```python
from build123d import *

# Parameters (mm, degrees)
EXTRUDE_1_DEPTH     = 3
SKETCH_2_R          = 1.6
SKETCH_2_W          = 1.5
SKETCH_2_H          = 40
CUT_EXTRUDE_1_DEPTH = 160.48040632


with BuildPart() as part:
    # 草图1 → 凸台-拉伸1 (new body)
    with BuildSketch(Plane.XY):
        Polygon((0, 0), (20, 0), (105, -105), (105, -120), (-20, -120), (-20, -105), align=None)
    extrude(amount=EXTRUDE_1_DEPTH)

    # 草图2 → 切除-拉伸1 (cut, through all)
    with BuildSketch(Plane.XY.offset(3)):
        with Locations((5, -5)):
            Circle(SKETCH_2_R)
        with Locations(Location((15, -5, 0), (0, 0, 180))):
            Circle(SKETCH_2_R)
        with Locations((15, -15)):
            Circle(SKETCH_2_R)
        with Locations(Location((5, -15, 0), (0, 0, 180))):
            Circle(SKETCH_2_R)
        with Locations((-15, -116.25)):
            Circle(SKETCH_2_R)
        with Locations(Location((-15, -108.75, 0), (0, 0, 180))):
            Circle(SKETCH_2_R)
        with Locations(Location((-5, -116.25, 0), (0, 0, 180))):
            Circle(SKETCH_2_R)
        with Locations((-5, -108.75)):
            Circle(SKETCH_2_R)
        with Locations(Location((90, -108.75, 0), (0, 0, 180))):
            Circle(SKETCH_2_R)
        with Locations((90, -116.25)):
            Circle(SKETCH_2_R)
        with Locations((100, -108.75)):
            Circle(SKETCH_2_R)
        with Locations(Location((100, -116.25, 0), (0, 0, 180))):
            Circle(SKETCH_2_R)
        with Locations((37.5, -116.25)):
            Circle(SKETCH_2_R)
        with Locations(Location((47.5, -116.25, 0), (0, 0, 180))):
            Circle(SKETCH_2_R)
        with Locations((47.5, -108.75)):
            Circle(SKETCH_2_R)
        with Locations(Location((37.5, -108.75, 0), (0, 0, 180))):
            Circle(SKETCH_2_R)
        with Locations((5, -45)):
            Circle(SKETCH_2_R)
        with Locations(Location((15, -45, 0), (0, 0, 180))):
            Circle(SKETCH_2_R)
        with Locations((15, -55)):
            Circle(SKETCH_2_R)
        with Locations(Location((5, -55, 0), (0, 0, 180))):
            Circle(SKETCH_2_R)
        with Locations(Location((5, -108.75, 0), (0, 0, 180))):
            Circle(SKETCH_2_R)
        with Locations((5, -116.25)):
            Circle(SKETCH_2_R)
        with Locations(Location((15, -116.25, 0), (0, 0, 180))):
            Circle(SKETCH_2_R)
        with Locations((15, -108.75)):
            Circle(SKETCH_2_R)
        with Locations((70, -116.25)):
            Circle(SKETCH_2_R)
        with Locations(Location((80, -116.25, 0), (0, 0, 180))):
            Circle(SKETCH_2_R)
        with Locations(Location((70, -108.75, 0), (0, 0, 180))):
            Circle(SKETCH_2_R)
        with Locations((80, -108.75)):
            Circle(SKETCH_2_R)
        Polygon((-2, -53.255116653), (-2, -102.5), (-11.37997778, -102.5), align=None)
        with Locations((104.25, -100)):
            Rectangle(SKETCH_2_W, SKETCH_2_H)
        with Locations((-19.25, -100)):
            Rectangle(SKETCH_2_W, SKETCH_2_H)
        Polygon((22, -34.257073144), (22, -102.5), (77.244274122, -102.5), align=None)
    extrude(amount=-CUT_EXTRUDE_1_DEPTH, mode=Mode.SUBTRACT)


solid = part.part
```
Geometry check sheet. Reference: the model listing, model coordinates, mm. A direction names the side the tool comes from. Round coordinates to 2 decimals unless told otherwise and drop trailing zeros. Order: outer loops, then holes, each group sorted by start corner. A loop starts at its lowest first (then second) coordinate and runs counter-clockwise, first axis right, second up. Notation, with made-up numbers: M 26,70 L 35,70 A27 cw 35,109 Z; hole C 60,-40 d6. An arc over 180 degrees is marked long. Answer as CSV lines item,"result".
1) Sectioned sample at A-A on x = 5. Record the cut outline in (y, z), and give its area (3 significant figures).
Entries:
outline,"M -120,0 L -117.85,0 L -117.85,3 L -120,3 Z; M -114.65,0 L -110.35,0 L -110.35,3 L -114.65,3 Z; M -107.15,0 L -56.6,0 L -56.6,3 L -107.15,3 Z; M -53.4,0 L -46.6,0 L -46.6,3 L -53.4,3 Z; M -43.4,0 L -16.6,0 L -16.6,3 L -43.4,3 Z; M -13.4,0 L -6.6,0 L -6.6,3 L -13.4,3 Z; M -3.4,0 L 0,0 L 0,3 L -3.4,3 Z"
area,"302 mm2"
2) Sectioned sample at D-D on y = -5. Record the cut outline in (x, z), and give its area (3 significant figures).
Entries:
outline,"M -0.95,0 L 3.4,0 L 3.4,3 L -0.95,3 Z; M 6.6,0 L 13.4,0 L 13.4,3 L 6.6,3 Z; M 16.6,0 L 24.05,0 L 24.05,3 L 16.6,3 Z"
area,"55.8 mm2"
3) Gauge pin test, flat ends, axial feed: pin 1 Ø4 at (x, y) = (90, -108.75) entering from +Z; pin 2 Ø1.5 at (x, z) = (82, 0.5) entering from +Y; pin 3 Ø0.9 at (y, z) = (-68.5, 2) entering from -X. Record the tip position at first contact, or that the pin passes through.
Entries:
pin 1,"z = 3"
pin 2,"y = -75.66"
pin 3,"x = -13.13"
4) Sectioned sample at C-C on x = 100. Record the cut outline in (y, z).
Entries:
outline,"M -120,0 L -117.85,0 L -117.85,3 L -120,3 Z; M -114.65,0 L -110.35,0 L -110.35,3 L -114.65,3 Z; M -107.15,0 L -98.82,0 L -98.82,3 L -107.15,3 Z"
5) Sectioned sample at B-B on y = -45. Record the cut outline in (x, z).
Entries:
outline,"M -8.57,0 L 3.4,0 L 3.4,3 L -8.57,3 Z; M 6.6,0 L 13.4,0 L 13.4,3 L 6.6,3 Z; M 16.6,0 L 22,0 L 22,3 L 16.6,3 Z; M 30.7,0 L 56.43,0 L 56.43,3 L 30.7,3 Z"
6) Thickness scan on probe 1 along X at (y, z) = (-77, 0.4); probe 2 along Y at (x, z) = (100, 1.55); probe 3 along X at (y, z) = (-70, 0.45). Record the ranges inside material, lowest first. Write a range as [from, to].
Entries:
probe 1,"[-14.67, -6.52], [-2, 22], [56.6, 82.33]"
probe 2,"[-120, -117.85], [-114.65, -110.35], [-107.15, -98.82]"
probe 3,"[-13.33, -5.19], [-2, 22], [50.93, 76.67]"
7) Tool access check on faces 1 (the face through (16, -72, 0)), 2 (the face through (49, -102.5, 2)). Record the directions out of +Z, -Z, +X, -X, +Y, -Y that give a thin tool (end or side, any length) a straight path to the whole face; none if there is none.
Entries:
face 1,"-Z, +X, -X, +Y, -Y"
face 2,"+Z, -Z"
8) Mould release check, pull along X, two halves, no side actions. Record for faces 3 (the face through (61.166, -50.852, 1.479)), 4 (the face through (10, 0, 1)), 5 (the face through (68.474, -109.231, 1.521)): +X half, -X half, draft (parallel to the pull), parting line (faces both ways), or undercut.
Entries:
face 3,"+X half"
face 4,"draft"
face 5,"undercut"
